Here's how the part is built. I have some questions about the finished solid (model axes, mm). Face numbers are marked on the shaded views. A direction names the side the tool comes from. Round coordinates to 2 decimals unless told otherwise and drop trailing zeros. Loops run counter-clockwise (first coordinate to the right, second up) from the corner with the lowest first, then second, coordinate; pieces in that order, holes last. Notation, with made-up numbers: (85.25, 1) - (138.25, 1) arc R15 cw to (138.25, 27) - close; hole circle Ø3 at (-13, -26). An arc over 180 degrees is marked (long way). Return JSON: item names as keys, results as strings. Group by question number.
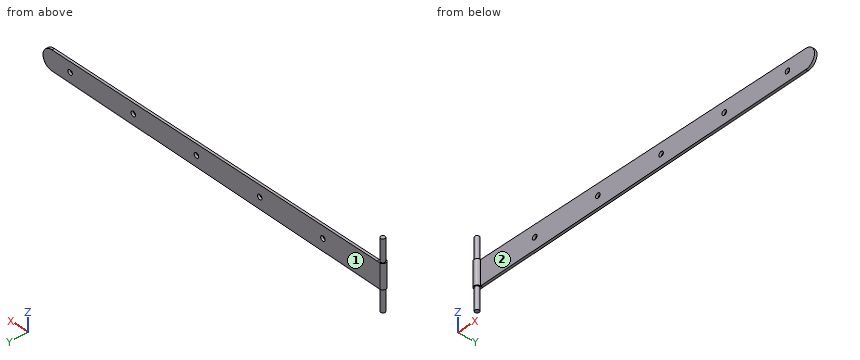
```python
from build123d import *

# Parameters (mm, degrees)
F1_DEPTH      = 6.35
F3_DEPTH      = 63.5
F5_R          = 5.55625
F6_DEPTH      = 88.9
F6_DEPTH_BACK = 88.9
F7_R          = 6.35
F8_DEPTH      = 6.35


with BuildPart() as f1:
    # F0 (on Front) → F1 (new body)
    with BuildSketch(Plane.XZ):
        with BuildLine():
            Line((914.5763676277, 57.1493876788), (0, 63.5))
            Line((0, 63.5), (0, 0))
            Line((0, 0), (914.5763676277, 6.3506123212))
            ThreePointArc((914.5763676277, 6.3506123212), (939.8, 31.75), (914.5763676277, 57.1493876788))
        make_face()
    extrude(amount=F1_DEPTH)

    # F2 (on Top) → F3 (join)
    with BuildSketch(Plane.XY):
        with BuildLine():
            Line((0, 0), (-7.7771299333, 0))
            ThreePointArc((-7.7771299333, 0), (-12.7972457189, -14.0858610621), (0, -6.35))
            Line((0, -6.35), (0, 0))
        make_face()
    extrude(amount=F3_DEPTH)

    # F5 (on mid) → F6 (join, two sides)
    with BuildSketch(Plane.XY.offset(31.75)) as f6_sk:
        with Locations((-7.7771299333, -7.9375)):
            Circle(F5_R)
    extrude(amount=F6_DEPTH)
    extrude(f6_sk.sketch, amount=-F6_DEPTH_BACK)

    # F7 (on face) → F8 (cut, through all)
    with BuildSketch(Plane.XZ.offset(6.35)):
        with Locations((152.4, 31.75)):
            Circle(F7_R)
        with Locations((330.2, 31.75)):
            Circle(F7_R)
        with Locations((508, 31.75)):
            Circle(F7_R)
        with Locations((685.8, 31.75)):
            Circle(F7_R)
        with Locations((863.6, 31.75)):
            Circle(F7_R)
    extrude(amount=-F8_DEPTH, mode=Mode.SUBTRACT)


solid = f1.part
```
Q1. Please list where these lines run through material, in increasing order: line 1 (Z direction, x = 508, y = -2.5); line 2 (Z direction, x = 685.8, y = -1.75); line 3 (Z direction, x = 304.5, y = -1.5).
Q2. Imagine slicing it at B-B, the plane z = -39.5. List the corners of the cut face in (x, y) for me, and give its area (3 significant figures).
Q3. Imagine slicing it at A-A, the plane x = 241.5. List the corners of the cut face in (y, z) for me.
Q4. Will these pins go through, and if not, where does the flat tip stop? pin 1 Ø1 at (y, z) = (-3.5, 37.5) entering from +X; pin 2 Ø14.5 at (x, z) = (508, 31.75) entering from -Y; pin 3 Ø10 at (x, z) = (152.4, 31.75) entering from -Y; pin 4 Ø1.5 at (y, z) = (-11.5, 18) entering from +X.
Q5. Imagine slicing it at C-C, the plane x = 759.5. List the corners of the cut face in (y, z) for me, and give its area (3 significant figures).
Q6. For the marked faces 1 and 2, which set-ups out of +Z, -Z, +X, -X, +Y, -Y let a thin tool reach every point of the face, with its end or its side?
Output values:
{
 "1": {"line 1": "z = 3.53 to 25.4, 38.1 to 59.97", "line 2": "z = 4.76 to 25.4, 38.1 to 58.74", "line 3": "z = 2.11 to 61.39"},
 "2": {"outline": "circle Ø11.11 at (-7.78, -7.94)", "area": "97.0 mm^2"},
 "3": {"outline": "(-6.35, 1.68) - (0, 1.68) - (0, 61.82) - (-6.35, 61.82) - close"},
 "4": {"pin 1": "stops at x = 939.25", "pin 2": "stops at y = -6.35", "pin 3": "passes through", "pin 4": "stops at x = -0.35"},
 "5": {"outline": "(-6.35, 5.27) - (0, 5.27) - (0, 58.23) - (-6.35, 58.23) - close", "area": "336 mm^2"},
 "6": {"face 1": "+Z, -Z, +X, -X, +Y", "face 2": "+Z, -Z, +X, -Y"}
}
